The model under review builds one solid part; all positions refer to its coordinate system, in mm. Face numbers are marked on the shaded views. A direction names the side the tool comes from. Coordinates: 2 decimals unless noted, no trailing zeros. Write each loop counter-clockwise with the first axis right and the second up, starting at its lowest first coordinate (ties: lowest second). Pieces come first, ordered by that corner, then holes. Notation, with made-up numbers: (60.25, 0) - (119.25, 0) arc R18 cw to (119.25, 16) - close; hole circle Ø2 at (28, 36.5). An arc over 180 degrees is marked (long way). Put each result on its own line as item: value. Start each with the question number.
Item 1: Consider section D-D on y = -41.5. Give the boundary of the cut face in (x, z).
Item 2: For pin 1 (5 mm diameter, centred on y = -29.5, z = 91.5, fed in from -X); pin 2 (4 mm diameter, centred on x = 99.5, y = -50.5, fed in from +Z); pin 3 (17.5 mm diameter, centred on y = -41, z = 142.5, fed in from +X), all flat-tipped, find the tip position at first contact; note any pin that passes through.
Item 3: Consider section A-A on y = -12. Give the boundary of the cut face in (x, z).
Item 4: Machinability: for the marked faces 1 and 2, which of the approach directions +Z, -Z, +X, -X, +Y, -Y give a long, thin tool a straight path to every point of the face, cutting with its end or side? Answer none if there is none.
Item 5: Consider section B-B on z = 313. Give the boundary of the cut face in (x, y).
Item 6: Consider section C-C on x = 100. Give the boundary of the cut face in (y, z).
Item 7: To check wall thickness, follow L1, parallel to Z at x = 87.5, y = -2; L2, parallel to Z at x = 97.5, y = -11; L3, parallel to X at y = -3.5, z = 287.5. State the ranges of each line that lie inside material, in increasing order. Write a range as [from, to].
Item 8: Mouldability with a two-part tool opening along Z and no side actions: class the marked faces 3 and 4 as pulls with the +Z half, pulls with the -Z half, needs draft (parallel to the pull), parting line crosses it, or undercut.
```python
from build123d import *

# Parameters (mm, degrees)
F0_W     = 304.8
F0_H     = 406.4
F0_W_2   = 254.0000006139
F0_H_2   = 355.6000006139
F1_DEPTH = 25.4
F2_W     = 304.8
F2_H     = 406.4
F3_DEPTH = 6.35
F5_DEPTH = 254.0000006139


with BuildPart() as f1:
    # F0 (on Front) → F1 (new body)
    with BuildSketch(Plane.XZ):
        with Locations((152.4, 203.2)):
            Rectangle(F0_W, F0_H)
        with Locations((152.4, 203.2)):
            Rectangle(F0_W_2, F0_H_2, mode=Mode.SUBTRACT)
    extrude(amount=F1_DEPTH)

    # F2 (on face) → F3 (join)
    with BuildSketch(Plane(origin=(0, 0, 0), x_dir=(-1, 0, 0), z_dir=(0, 1, 0))):
        with Locations((-152.4, 203.2)):
            Rectangle(F2_W, F2_H)
    extrude(amount=F3_DEPTH)

    # F4 (on face) → F5 (join, through all)
    with BuildSketch(Plane.YZ.offset(25.399999693)):
        Polygon((-64.1043111682, 129.9178004265), (-25.4, 129.9178004265), (-25.4, 136.2678004265), (-57.7543111682, 136.2678004265), (-57.7543111682, 165.3573513031), (-64.1043111682, 165.3573513031), align=None)
        Polygon((0, 129.9178004265), (0, 271.2446153164), (-6.35, 271.2446153164), (-6.35, 136.2678004265), (-25.4, 136.2678004265), (-25.4, 129.9178004265), align=None)
    extrude(amount=F5_DEPTH)


solid = f1.part
```
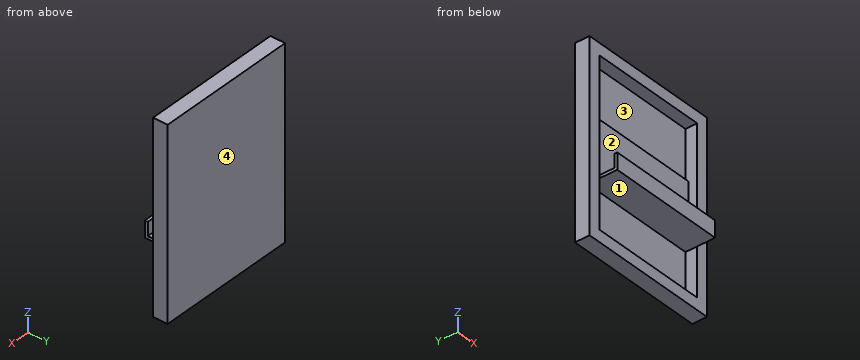
Report:
1. outline: (25.4, 129.92) - (279.4, 129.92) - (279.4, 136.27) - (25.4, 136.27) - close
2. pin 1: through
2. pin 2: z = 136.27
2. pin 3: x = 279.4
3. outline: (0, 0) - (304.8, 0) - (304.8, 406.4) - (0, 406.4) - close; hole (25.4, 25.4) - (279.4, 25.4) - (279.4, 129.92) - (25.4, 129.92) - close; hole (25.4, 136.27) - (279.4, 136.27) - (279.4, 381) - (25.4, 381) - close
4. face 1: -Y
4. face 2: none
5. outline: (0, -25.4) - (25.4, -25.4) - (25.4, 0) - (279.4, 0) - (279.4, -25.4) - (304.8, -25.4) - (304.8, 6.35) - (0, 6.35) - close
6. outline: (-64.1, 129.92) - (0, 129.92) - (0, 25.4) - (-25.4, 25.4) - (-25.4, 0) - (6.35, 0) - (6.35, 406.4) - (-25.4, 406.4) - (-25.4, 381) - (0, 381) - (0, 271.24) - (-6.35, 271.24) - (-6.35, 136.27) - (-57.75, 136.27) - (-57.75, 165.36) - (-64.1, 165.36) - close
7. L1: [0, 25.4], [129.92, 271.24], [381, 406.4]
7. L2: [0, 25.4], [129.92, 136.27], [381, 406.4]
7. L3: [0, 25.4], [279.4, 304.8]
8. face 3: undercut
8. face 4: needs draft
